Geometry: final body of the model. Coordinates: model frame, mm. Face numbers are marked on the shaded views. A direction names the side the tool comes from. Round coordinates to 2 decimals unless told otherwise and drop trailing zeros. Loops run counter-clockwise (first coordinate to the right, second up) from the corner with the lowest first, then second, coordinate; pieces in that order, holes last. Notation, with made-up numbers: (23, 8.5) - (52, 8.5) arc R10 ccw to (52, 18.5) - close; hole circle Ø1 at (56, 60). An arc over 180 degrees is marked (long way). Answer as a JSON object with one key per item and string values. Group by question number.
Item 1: Draft query along Y for the marked faces 3, 4, 5 and 6. Return one class per face: released by +Y, released by -Y, zero draft, split by the parting line, or undercut.
Item 2: Section A-A (x = 38.1). Return the cut outline in (y, z), plus the area to 3 significant figures.
Item 3: Section B-B (z = 2.25). Count the separate pieces of the cut face and the enclosed holes in it, plus the area to 3 significant figures.
Item 4: Reachability of the marked faces 1 and 2 from +Z, -Z, +X, -X, +Y, -Y: full face, straight path, thin tool, end or side. Return the list, or none.
Item 5: Section D-D (y = 2.5). Return the cut outline in (x, z) (3 decimals).
Item 6: First-contact query: pin 1 (2.5 mm diameter, centred on x = 3.175, z = 3.175, fed in from +Y); pin 2 (3 mm diameter, centred on x = 2.5, z = 3, fed in from +Y); pin 3 (1 mm diameter, centred on x = 30.5, z = 1, fed in from +Y). Flat tips, straight axial feed; report the tip coordinate or a pass-through.
Item 7: Line query: line 1 (X direction, y = 9.25, z = 5.5); line 2 (X direction, y = 7.25, z = 0.5); line 3 (X direction, y = 3.5, z = 3) (3 decimals). Output: solid intervals per line, ascending.
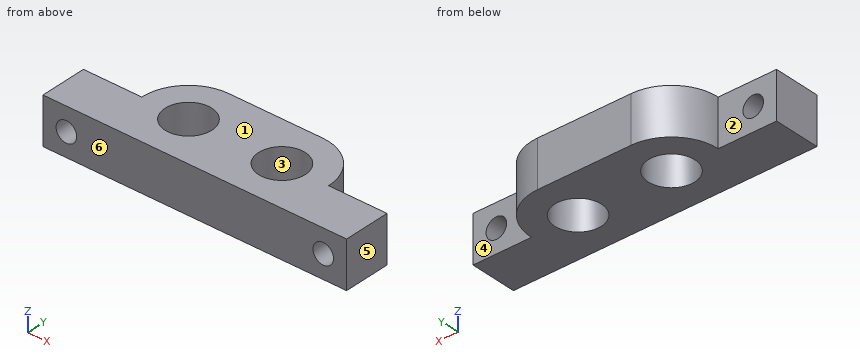
```python
from build123d import *

# Parameters (mm, degrees)
SKETCH1_R           = 3.175
BOSS_EXTRUDE1_DEPTH = 6.35
CUT_EXTRUDE1_REACH  = 8.35
SKETCH2_R           = 1.397


with BuildPart() as part:
    # Sketch1 → Boss-Extrude1 (new body)
    with BuildSketch(Plane.XY):
        with BuildLine():
            Line((0, 0), (41.275, 0))
            Line((41.275, 0), (41.275, 6.35))
            Line((41.275, 6.35), (33.3375, 6.35))
            ThreePointArc((33.3375, 6.35), (31.477628061, 10.840128061), (26.9875, 12.7))
            Line((26.9875, 12.7), (14.2875, 12.7))
            ThreePointArc((14.2875, 12.7), (9.797371939, 10.840128061), (7.9375, 6.35))
            Line((7.9375, 6.35), (0, 6.35))
            Line((0, 6.35), (0, 0))
        make_face()
        with Locations((14.2875, 6.35)):
            Circle(SKETCH1_R, mode=Mode.SUBTRACT)
        with Locations((26.9875, 6.35)):
            Circle(SKETCH1_R, mode=Mode.SUBTRACT)
    extrude(amount=BOSS_EXTRUDE1_DEPTH)

    # Sketch2 → Cut-Extrude1 (cut, up to next)
    with BuildSketch(Plane(origin=(0, 6.35, 0), x_dir=(1, 0, 0), z_dir=(0, 1, 0)), mode=Mode.PRIVATE) as cut_extrude1_sk1:
        with Locations((38.1, -3.175)):
            Circle(SKETCH2_R)
    cut_extrude1_tool1 = extrude(cut_extrude1_sk1.sketch, amount=-CUT_EXTRUDE1_REACH, mode=Mode.PRIVATE) & part.part
    add(cut_extrude1_tool1.solids().sort_by_distance((38.1, 6.35, 3.175))[0], mode=Mode.SUBTRACT)
    # Sketch2 → Cut-Extrude1 (cut, up to next)
    with BuildSketch(Plane(origin=(0, 6.35, 0), x_dir=(1, 0, 0), z_dir=(0, 1, 0)), mode=Mode.PRIVATE) as cut_extrude1_sk2:
        with Locations((3.175, -3.175)):
            Circle(SKETCH2_R)
    cut_extrude1_tool2 = extrude(cut_extrude1_sk2.sketch, amount=-CUT_EXTRUDE1_REACH, mode=Mode.PRIVATE) & part.part
    add(cut_extrude1_tool2.solids().sort_by_distance((3.175, 6.35, 3.175))[0], mode=Mode.SUBTRACT)


solid = part.part
```
Values:
{
 "1": {"face 3": "undercut", "face 4": "released by +Y", "face 5": "zero draft", "face 6": "released by -Y"},
 "2": {"outline": "(0, 0) - (6.35, 0) - (6.35, 1.78) - (0, 1.78) - close; (0, 4.57) - (6.35, 4.57) - (6.35, 6.35) - (0, 6.35) - close", "area": "22.6 mm^2"},
 "3": {"separate pieces": "3", "enclosed holes": "2", "area": "316 mm^2"},
 "4": {"face 1": "+Z, +X, -X, +Y, -Y", "face 2": "+Z, -Z, -X, +Y"},
 "5": {"outline": "(0, 0) - (41.275, 0) - (41.275, 6.35) - (0, 6.35) - close; hole circle Ø2.794 at (3.175, 3.175); hole circle Ø2.794 at (38.1, 3.175)"},
 "6": {"pin 1": "passes through", "pin 2": "stops at y = 6.35", "pin 3": "stops at y = 11.94"},
 "7": {"line 1": "x = 8.64 to 12.99, 15.58 to 25.69, 28.28 to 32.64", "line 2": "x = 8 to 11.24, 17.33 to 23.94, 30.03 to 33.27", "line 3": "x = 0 to 1.789, 4.561 to 12.888, 15.687 to 25.588, 28.387 to 36.714, 39.486 to 41.275"}
}
